```python
from build123d import *

# Parameters (mm, degrees)
SKETCH1_R           = 6.5
SKETCH1_R_2         = 2.5
BOSS_EXTRUDE1_DEPTH = 2
SKETCH2_R           = 5.5
SKETCH2_R_2         = 3.5
BOSS_EXTRUDE2_DEPTH = 90
BOSS_EXTRUDE3_START = -2
SKETCH4_R           = 3.5
BOSS_EXTRUDE3_DEPTH = 2
SKETCH5_R           = 12.5
BOSS_EXTRUDE4_DEPTH = 2
SKETCH6_R           = 2.1
CUT_EXTRUDE1_DEPTH  = 10


with BuildPart() as part:
    # Sketch1 → Boss-Extrude1 (new body)
    with BuildSketch(Plane.XY):
        Circle(SKETCH1_R)
        Circle(SKETCH1_R_2, mode=Mode.SUBTRACT)
    extrude(amount=BOSS_EXTRUDE1_DEPTH)

    # Sketch2 → Boss-Extrude2 (add)
    with BuildSketch(Plane.XY.offset(2)):
        with Locations(Location((0, 0, 0), (0, 0, 180))):
            Circle(SKETCH2_R)
        with Locations(Location((0, 0, 0), (0, 0, 180))):
            Circle(SKETCH2_R_2, mode=Mode.SUBTRACT)
    extrude(amount=BOSS_EXTRUDE2_DEPTH)

    # Sketch4 → Boss-Extrude3 (add)
    with BuildSketch(Plane.XY.offset(92).offset(BOSS_EXTRUDE3_START)):
        with Locations(Location((0, 0, 0), (0, 0, 180))):
            Circle(SKETCH4_R)
    extrude(amount=BOSS_EXTRUDE3_DEPTH)

    # Sketch5 → Boss-Extrude4 (add)
    with BuildSketch(Plane.XY.offset(92)):
        Circle(SKETCH5_R)
    extrude(amount=BOSS_EXTRUDE4_DEPTH)

    # Sketch6 → Cut-Extrude1 (cut)
    with BuildSketch(Plane(origin=(0, 0, 92), x_dir=(-1, 0, 0), z_dir=(0, 0, -1))):
        with Locations((0, 9)):
            Circle(SKETCH6_R)
        with Locations((9, 0)):
            Circle(SKETCH6_R)
        with Locations((0, -9)):
            Circle(SKETCH6_R)
        with Locations((-9, 0)):
            Circle(SKETCH6_R)
    extrude(amount=-CUT_EXTRUDE1_DEPTH, mode=Mode.SUBTRACT)


solid = part.part
```
The model under review builds one solid part; all positions refer to its coordinate system, in mm. A direction names the side the tool comes from. Give positions to 0.01 mm unless a question says otherwise; leave off trailing zeros. Loops run counter-clockwise (first coordinate to the right, second up) from the corner with the lowest first, then second, coordinate; pieces in that order, holes last. Notation, with made-up numbers: (88, 59.25) -> (137, 59.25) arc R17 cw to (137, 68.25) -> close; hole circle Ø4 at (57.25, -27.5). An arc over 180 degrees is marked (long way). Use CSV: the item, a comma, the result in double quotes.
1. To check wall thickness, follow probe 1 along Y at (x, z) = (0, 93.2); probe 2 along Z at (x, y) = (-3, 0.5); probe 3 along Z at (x, y) = (-7, 9.25). State the ranges of each line that lie inside material, in increasing order. Write a range as from..to.
Result:
probe 1,"y = -12.5..-11.1, -6.9..6.9, 11.1..12.5"
probe 2,"z = 0..2, 90..94"
probe 3,"z = 92..94"
2. The part is to be moulded in two halves that separate along X. For faces 1 (the face through (0, 0, 94)), 2 (the face through (11.923, 3.755, 92.986)), 3 (the face through (0.273, -6.918, 92.986)), say which applies: +X half, -X half, draft (parallel to the pull), parting line (faces both ways), or undercut.
Result:
face 1,"draft"
face 2,"parting line"
face 3,"undercut"
3. Consider section A-A, the plane y = 0. Write out the cut boundary in (x, z), then the cut area to 3 significant figures.
Result:
outline,"(-12.5, 92) -> (-11.1, 92) -> (-11.1, 94) -> (-12.5, 94) -> close; (-6.9, 92) -> (-5.5, 92) -> (-5.5, 2) -> (-6.5, 2) -> (-6.5, 0) -> (-2.5, 0) -> (-2.5, 2) -> (-3.5, 2) -> (-3.5, 90) -> (3.5, 90) -> (3.5, 2) -> (2.5, 2) -> (2.5, 0) -> (6.5, 0) -> (6.5, 2) -> (5.5, 2) -> (5.5, 92) -> (6.9, 92) -> (6.9, 94) -> (-6.9, 94) -> close; (11.1, 92) -> (12.5, 92) -> (12.5, 94) -> (11.1, 94) -> close"
area,"423 mm²"
4. Consider section B-B, the plane x = 9. Write out the cut boundary in (y, z).
Result:
outline,"(-8.67, 92) -> (-2.1, 92) -> (-2.1, 94) -> (-8.67, 94) -> close; (2.1, 92) -> (8.67, 92) -> (8.67, 94) -> (2.1, 94) -> close"
5. Machinability: for faces 4 (the face through (-5, 3, 2)), 5 (the face through (-6.9, 0.09, 92.99)), 6 (the face through (-5.158, -3.955, 0.986)), which of the approach directions +Z, -Z, +X, -X, +Y, -Y give a long, thin tool a straight path to every point of the face, cutting with its end or side? Answer none if there is none.
Result:
face 4,"none"
face 5,"+Z, -Z"
face 6,"-Z"
6. For P1, Ø2.5, axis at x = 0, y = 9, coming from the -Z side; P2, Ø12, axis at x = -5, z = 15.5, coming from the +Y side; P3, Ø2, axis at x = 0.5, z = 71, coming from the -Y side; P4, Ø10, axis at y = 8, z = 69, coming from the -X side, all flat-tipped, find the tip position at first contact; note any pin that passes through.
Result:
P1,"passes through"
P2,"stops at y = 5.5"
P3,"stops at y = -5.5"
P4,"stops at x = -4.61"
